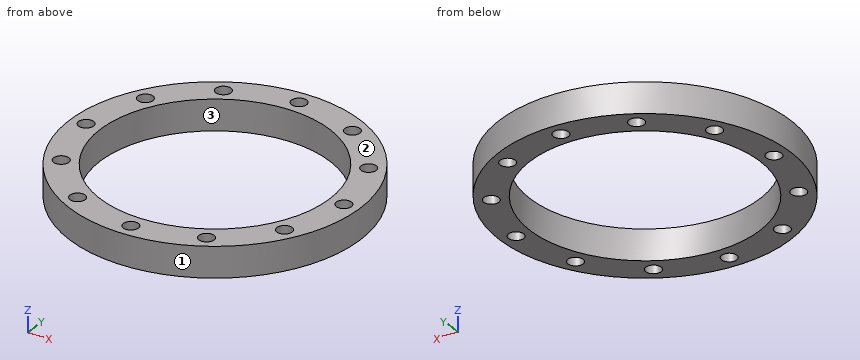
```python
from build123d import *

# Parameters (mm, degrees)
SKETCH1_R              = 241.3
SKETCH1_R_2            = 190.5
BOSS_EXTRUDE1_DEPTH    = 25.4
F_1_1_DIAMETER_HOLE1_D = 25.4
CIRPATTERN1_COUNT      = 12


with BuildPart() as part:
    # Sketch1 → Boss-Extrude1 (new body, symmetric)
    with BuildSketch(Plane.XY):
        Circle(SKETCH1_R)
        Circle(SKETCH1_R_2, mode=Mode.SUBTRACT)
    extrude(amount=BOSS_EXTRUDE1_DEPTH, both=True)

    # 1 (1) Diameter Hole1 (through all)
    with Locations(Plane.XY.offset(25.4)):
        with Locations((215.9, 0)):
            f_1_1_diameter_hole1 = Hole(F_1_1_DIAMETER_HOLE1_D / 2)

    # CirPattern1: 1 (1) Diameter Hole1 ×12 about axis
    cirpattern1_axis = Axis((0, 0, 0), (0, 0, 1))
    for i in range(1, CIRPATTERN1_COUNT):
        add(f_1_1_diameter_hole1.rotate(cirpattern1_axis, i * 360 / CIRPATTERN1_COUNT), mode=Mode.SUBTRACT)


solid = part.part
```
The model under review builds one solid part; all positions refer to its coordinate system, in mm. Face numbers are marked on the shaded views. Round coordinates to 2 decimals unless told otherwise and drop trailing zeros. Write each loop counter-clockwise with the first axis right and the second up, starting at its lowest first coordinate (ties: lowest second). Pieces come first, ordered by that corner, then holes. Notation, with made-up numbers: (-23, 18.5) - (-17, 18.5) arc R32 cw to (-17, 50.5) - close; hole circle Ø6 at (3.5, 51.5). An arc over 180 degrees is marked (long way). Answer as CSV lines item,"result". Start each with the question number.
(1) We need section C-C on y = 211. State the section outline as (x, z) points, plus the area to 3 significant figures.
(2) Draft analysis for pull direction Y (two halves, no side actions). For the marked faces 1, 2 and 3, state which applies: pulls with the +Y half, pulls with the -Y half, needs draft (parallel to the pull), parting line crosses it, or undercut.
(3) We need section B-B on x = -215.9. State the section outline as (y, z) points.
(4) For pin 1 Ø8 at (x, z) = (-34, -15.5) entering from -Y; pin 2 Ø1.5 at (y, z) = (48, 8) entering from -X; pin 3 Ø10 at (x, z) = (-117.5, 3.5) entering from +Y; pin 4 Ø12 at (y, z) = (-0.5, -10) entering from -X, all flat-tipped, find the tip position at first contact; note any pin that passes through.
(5) We need section D-D on x = 107.95. State the section outline as (y, z) points, plus the area to 3 significant figures.
(6) To check wall thickness, follow line 1 (Y direction, x = 1, z = -17); line 2 (Y direction, x = 196, z = -21.5); line 3 (Y direction, x = -18, z = -12). State the ranges of each line that lie inside material, in increasing order.
(7) We need section A-A on y = 0. State the section outline as (x, z) points, plus the area to 3 significant figures.
Worked answers:
1,outline,"(-117.07, -25.4) - (-11.72, -25.4) - (-11.72, 25.4) - (-117.07, 25.4) - close; (11.72, -25.4) - (117.07, -25.4) - (117.07, 25.4) - (11.72, 25.4) - close"
1,area,"10,700 mm²"
2,face 1,"parting line crosses it"
2,face 2,"needs draft"
2,face 3,"undercut"
3,outline,"(-107.76, -25.4) - (-12.7, -25.4) - (-12.7, 25.4) - (-107.76, 25.4) - close; (12.7, -25.4) - (107.76, -25.4) - (107.76, 25.4) - (12.7, 25.4) - close"
4,pin 1,"y = -239.43"
4,pin 2,"x = -236.63"
4,pin 3,"y = 213.47"
4,pin 4,"x = -241.3"
5,outline,"(-215.81, -25.4) - (-199.67, -25.4) - (-199.67, 25.4) - (-215.81, 25.4) - close; (-174.27, -25.4) - (-156.96, -25.4) - (-156.96, 25.4) - (-174.27, 25.4) - close; (156.96, -25.4) - (174.27, -25.4) - (174.27, 25.4) - (156.96, 25.4) - close; (199.67, -25.4) - (215.81, -25.4) - (215.81, 25.4) - (199.67, 25.4) - close"
5,area,"3,400 mm²"
6,line 1,"-241.3 to -228.56, -203.24 to -190.5, 190.5 to 203.24, 228.56 to 241.3"
6,line 2,"-140.75 to -116.89, -99.01 to 99.01, 116.89 to 140.75"
6,line 3,"-240.63 to -189.65, 189.65 to 240.63"
7,outline,"(-241.3, -25.4) - (-228.6, -25.4) - (-228.6, 25.4) - (-241.3, 25.4) - close; (-203.2, -25.4) - (-190.5, -25.4) - (-190.5, 25.4) - (-203.2, 25.4) - close; (190.5, -25.4) - (203.2, -25.4) - (203.2, 25.4) - (190.5, 25.4) - close; (228.6, -25.4) - (241.3, -25.4) - (241.3, 25.4) - (228.6, 25.4) - close"
7,area,"2,580 mm²"
